```python
from build123d import *

# Parameters (mm, degrees)
BOSS_EXTRUDE1_DEPTH = 15
SKETCH2_W           = 3
SKETCH2_H           = 41.822305452
CUT_EXTRUDE1_DEPTH  = 12
CHAMFER1_SIZE       = 1
SKETCH3_W           = 5.696125243
SKETCH3_H           = 11.031228464
CUT_EXTRUDE2_DEPTH  = 22


with BuildPart() as part:
    # Sketch1 → Boss-Extrude1 (new body)
    with BuildSketch(Plane(origin=(0, 0, 0), x_dir=(1, 0, 0), z_dir=(0, 1, 0))):
        Polygon((0, 0), (5, 0), (5, 19), (-6, 19), (-6, -6), (5, -6), (5, -3), (0, -3), align=None)
    extrude(amount=BOSS_EXTRUDE1_DEPTH)

    # Sketch2 → Cut-Extrude1 (cut)
    with BuildSketch(Plane.XZ):
        with Locations((-1.5, -17.911152726)):
            Rectangle(SKETCH2_W, SKETCH2_H)
    extrude(amount=-CUT_EXTRUDE1_DEPTH, mode=Mode.SUBTRACT)

    # Chamfer1
    chamfer1_edges = [part.edges().sort_by_distance(p)[0] for p in [
        (-6, 7.5, 6),
        (-6, 15, -6.5),
        (-0.5, 15, 6),
    ]]
    chamfer(chamfer1_edges, length=CHAMFER1_SIZE)

    # Sketch3 → Cut-Extrude2 (cut)
    with BuildSketch(Plane(origin=(0, 0, -19), x_dir=(-1, 0, 0), z_dir=(0, 0, -1))):
        with Locations((-2.848062622, 1.484385768)):
            Rectangle(SKETCH3_W, SKETCH3_H)
    extrude(amount=-CUT_EXTRUDE2_DEPTH, mode=Mode.SUBTRACT)


solid = part.part
```
Geometry: final body of the model. Coordinates: model frame, mm. A direction names the side the tool comes from. Give positions to 0.01 mm unless a question says otherwise; leave off trailing zeros. Loops run counter-clockwise (first coordinate to the right, second up) from the corner with the lowest first, then second, coordinate; pieces in that order, holes last. Notation, with made-up numbers: (-25, 16.5) -> (-11, 16.5) arc R26 ccw to (-11, 36.5) -> close; hole circle Ø1 at (33, -12.75). An arc over 180 degrees is marked (long way). Return JSON: item names as keys, results as strings.
Item 1: Access query for faces 5 (the flat face through (1, 9, -19)), 6 (the flat face through (3, 7, -10)), 7 (the flat face through (0, 9, -10)), 8 (the flat face through (1, 7, 3)), 9 (the flat face through (-4, 0, -4)). Directions: +Z, -Z, +X, -X, +Y, -Y. A direction counts if a zero-diameter tool reaches every point of the face in a straight line with its end or side. Return the directions, or none.
Filled in:
{"face 5": "-Z, +X, -X, +Y, -Y", "face 6": "-Z, +X, -Y", "face 7": "-Z, -Y", "face 8": "+X, -Y", "face 9": "+Z, -Z, +X, -X, -Y"}
Item 2: Section C-C, the plane x = -2.75. Output: boundary loops of the cut face in (y, z).
Filled in:
{"outline": "(0, 3) -> (12, 3) -> (12, -19) -> (15, -19) -> (15, 5) -> (14, 6) -> (0, 6) -> close"}
Item 3: Section B-B, the plane y = 10. Output: boundary loops of the cut face in (x, z).
Filled in:
{"outline": "(-6, -19) -> (-3, -19) -> (-3, 3) -> (5, 3) -> (5, 6) -> (-5, 6) -> (-6, 5) -> close; (0, -19) -> (5, -19) -> (5, 0) -> (0, 0) -> close"}
Item 4: Mould query, pull axis X, two halves, no side actions, for faces 1 (the flat face through (-2, 12, -8)), 2 (the flat face through (-6, 7, -7)), 3 (the flat face through (0, 13, 2)), 4 (the flat face through (2, 11, 0)). Classes: released by +X, released by -X, zero draft, split by the parting line, or undercut.
Filled in:
{"face 1": "undercut", "face 2": "released by -X", "face 3": "released by +X", "face 4": "zero draft"}
Item 5: Section A-A, the plane x = 0.25. Output: boundary loops of the cut face in (y, z).
Filled in:
{"outline": "(0, 3) -> (15, 3) -> (15, 5) -> (14, 6) -> (0, 6) -> close; (7, -19) -> (15, -19) -> (15, 0) -> (7, 0) -> close"}
Item 6: Section D-D, the plane z = -9.75. Output: boundary loops of the cut face in (x, y), plus the area to 3 significant figures.
Filled in:
{"outline": "(-6, 0) -> (-3, 0) -> (-3, 12) -> (0, 12) -> (0, 7) -> (5, 7) -> (5, 15) -> (-5, 15) -> (-6, 14) -> close", "area": "93.5 mm^2"}
Item 7: Pin query (flat end, axial travel): P1, Ø2.5, axis at y = 13.5, z = 1.5, coming from the +X side; P2, Ø4, axis at x = 3, z = -13.5, coming from the -Y side. Return the tip coordinate at first contact, or that it passes through.
Filled in:
{"P1": "x = 0", "P2": "y = 7"}
Item 8: Line query: line 1 (Z direction, x = 1.25, y = 6.25); line 2 (Z direction, x = 2.25, y = 10.5); line 3 (X direction, y = 1.25, z = 0). Output: solid intervals per line, ascending.
Filled in:
{"line 1": "3 to 6", "line 2": "-19 to 0, 3 to 6", "line 3": "-6 to -3"}
